Answer from the drawing. Dimensions are ordinates in mm from the lowest x, y and z of the part. Give positions to 0.01 mm unless a question says otherwise; leave off trailing zeros. Order: outer loops, then holes, each group sorted by start corner. A loop starts at its lowest first (then second) coordinate and runs counter-clockwise, first axis right, second up.
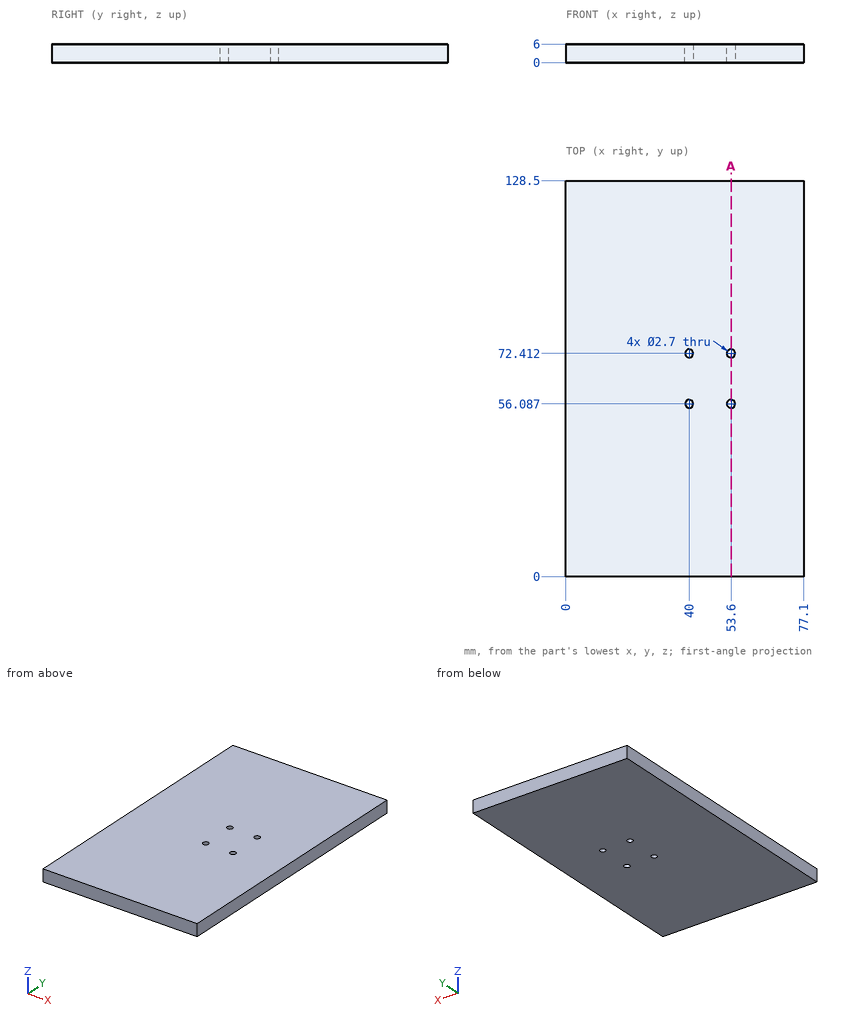
1. Straight lines are drawn through the part: probe 1 along Y at (x, z) = (40, 3.45); probe 2 along X at (y, z) = (57, 1.85) (1 decimal). For each, find the intervals that lie inside material, in ascending order.
Findings below:
probe 1: y = 0 to 54.74, 57.44 to 71.06, 73.76 to 128.5
probe 2: x = 0 to 39, 41 to 52.6, 54.6 to 77.1
2. Given P1, Ø2.5, axis at x = 53.6, y = 56.09, coming from the +Z side; P2, Ø1.5, axis at x = 50.5, y = 50, coming from the -Z side, each flat-ended and moving along its own axis, determine where each tip first touches the part or whether it passes through.
Findings below:
P1: passes through
P2: stops at z = 0
3. The part is cut by section A-A (x = 53.6). Write down the section's boundary in (y, z).
Findings below:
outline: (0, 0) - (54.74, 0) - (54.74, 6) - (0, 6) - close; (57.44, 0) - (71.06, 0) - (71.06, 6) - (57.44, 6) - close; (73.76, 0) - (128.5, 0) - (128.5, 6) - (73.76, 6) - close
